from build123d import *

# Parameters (mm, degrees)
SKETCH1_W           = 85
SKETCH1_H           = 115
BOSS_EXTRUDE1_DEPTH = 3
SKETCH2_R           = 1.6
CUT_EXTRUDE1_DEPTH  = 40


with BuildPart() as part:
    # Sketch1 → Boss-Extrude1 (new body)
    with BuildSketch(Plane(origin=(0, 0, 0), x_dir=(1, 0, 0), z_dir=(0, 1, 0))):
        Rectangle(SKETCH1_W, SKETCH1_H)
        with BuildLine():
            Line((-36.5, -57.5), (-42.5, -57.5))
            Line((-42.5, -57.5), (-42.5, -51.5))
            ThreePointArc((-42.5, -51.5), (-46.742640687, -61.742640687), (-36.5, -57.5))
        make_face()
        with BuildLine():
            Line((42.5, -57.5), (36.5, -57.5))
            ThreePointArc((36.5, -57.5), (46.742640687, -61.742640687), (42.5, -51.5))
            Line((42.5, -51.5), (42.5, -57.5))
        make_face()
        with BuildLine():
            Line((42.5, 57.5), (42.5, 51.5))
            ThreePointArc((42.5, 51.5), (46.742640687, 61.742640687), (36.5, 57.5))
            Line((36.5, 57.5), (42.5, 57.5))
        make_face()
        with BuildLine():
            ThreePointArc((-36.5, 57.5), (-46.742640687, 61.742640687), (-42.5, 51.5))
            Line((-42.5, 51.5), (-42.5, 57.5))
            Line((-42.5, 57.5), (-36.5, 57.5))
        make_face()
    extrude(amount=BOSS_EXTRUDE1_DEPTH)

    # Sketch2 → Cut-Extrude1 (cut)
    with BuildSketch(Plane.XZ):
        with Locations((-42.5, 57.5)):
            Circle(SKETCH2_R)
        with Locations((42.5, 57.5)):
            Circle(SKETCH2_R)
        with Locations((42.5, -57.5)):
            Circle(SKETCH2_R)
        with Locations((-42.5, -57.5)):
            Circle(SKETCH2_R)
    extrude(amount=-CUT_EXTRUDE1_DEPTH, mode=Mode.SUBTRACT)


solid = part.part
Read the model definition and answer for the solid it produces. Units are mm, in the model's axes. A direction names the side the tool comes from. Give positions to 0.01 mm unless a question says otherwise; leave off trailing zeros. Write each loop counter-clockwise with the first axis right and the second up, starting at its lowest first coordinate (ties: lowest second). Pieces come first, ordered by that corner, then holes. Notation, with made-up numbers: (-19, 30) - (-13, 30) arc R30 ccw to (-13, 52) - close; hole circle Ø3 at (-3.5, 48). An arc over 180 degrees is marked (long way). Answer in a Markdown table with one row per item. Add a question column.
Item 1: A tool of negligible diameter and unlimited length cuts with its end or side. For faces 4 (the face through (-46.6, 1.48, -61.88)), 5 (the face through (42.5, 1, 1)), 6 (the face through (-1, 1, -57.5)), 7 (the face through (-1, 1, 57.5)), from which of +Z, -Z, +X, -X, +Y, -Y can it reach the whole face along a straight path? Write none if from no direction.
Item 2: Section C-C, the plane z = 12 is taken. Write down the section's boundary in (x, y), and give its area (3 significant figures).
Item 3: Determine the mould class of faces 1 (the face through (-42.5, 1, 1)), 2 (the face through (42.292, 1.479, 59.086)), 3 (the face through (-1, 3, -1)) for opening direction X: pulls with the +X half, pulls with the -X half, needs draft (parallel to the pull), parting line crosses it, or undercut.
Item 4: Section A-A, the plane y = 1.95 is taken. Write down the section's boundary in (x, z).
Item 5: Section B-B, the plane x = 22 is taken. Write down the section's boundary in (y, z), and give its area (3 significant figures).
Item 6: Find the intervals of material crossed by L1, parallel to Z at x = 6, y = 2.9; L2, parallel to X at y = 1.15, z = -8, in increasing order.
Item 7: Flat-ended cylindrical pins translate along their axes: P1, Ø0.9, axis at x = 10, y = 1.5, coming from the +Z side; P2, Ø1.5, axis at x = -19.5, y = 0.5, coming from the -Z side; P3, Ø0.9, axis at y = 1, z = -9.5, coming from the -X side. Find the tip coordinate at first contact, or state that the pin passes through.
Recorded:
| question | item | result |
|---|---|---|
| 1 | face 4 | +Y, -Y |
| 1 | face 5 | +X, +Y, -Y |
| 1 | face 6 | -Z, +Y, -Y |
| 1 | face 7 | +Z, +Y, -Y |
| 2 | outline | (-42.5, 0) - (42.5, 0) - (42.5, 3) - (-42.5, 3) - close |
| 2 | area | 255 mm2 |
| 3 | face 1 | pulls with the -X half |
| 3 | face 2 | undercut |
| 3 | face 3 | needs draft |
| 4 | outline | (-42.5, -51.5) arc R6 ccw (long way) to (-36.5, -57.5) - (36.5, -57.5) arc R6 ccw (long way) to (42.5, -51.5) - (42.5, 51.5) arc R6 ccw (long way) to (36.5, 57.5) - (-36.5, 57.5) arc R6 ccw (long way) to (-42.5, 51.5) - close; hole circle Ø3.2 at (-42.5, -57.5); hole circle Ø3.2 at (-42.5, 57.5); hole circle Ø3.2 at (42.5, -57.5); hole circle Ø3.2 at (42.5, 57.5) |
| 5 | outline | (0, -57.5) - (3, -57.5) - (3, 57.5) - (0, 57.5) - close |
| 5 | area | 345 mm2 |
| 6 | L1 | z = -57.5 to 57.5 |
| 6 | L2 | x = -42.5 to 42.5 |
| 7 | P1 | stops at z = 57.5 |
| 7 | P2 | stops at z = -57.5 |
| 7 | P3 | stops at x = -42.5 |
